from build123d import *

# Parameters (mm, degrees)
ESQUISSE1_W        = 400
ESQUISSE1_H        = 100
ESQUISSE1_W_2      = 395
ESQUISSE1_H_2      = 95
BOSS_EXTRU_2_DEPTH = 100
ESQUISSE3_W        = 400
ESQUISSE3_H        = 100
ESQUISSE3_W_2      = 380
ESQUISSE3_H_2      = 80
BOSS_EXTRU_3_DEPTH = 25
BOSS_EXTRU_4_START = 100
ESQUISSE4_W        = 70
ESQUISSE4_H        = 25
ESQUISSE4_W_2      = 25
ESQUISSE4_H_2      = 70
BOSS_EXTRU_4_DEPTH = 10


with BuildPart() as part:
    # Esquisse1 → Boss.-Extru.2 (new body)
    with BuildSketch(Plane.XY):
        Rectangle(ESQUISSE1_W, ESQUISSE1_H)
        Rectangle(ESQUISSE1_W_2, ESQUISSE1_H_2, mode=Mode.SUBTRACT)
    extrude(amount=BOSS_EXTRU_2_DEPTH)

    # Esquisse3 → Boss.-Extru.3 (add)
    with BuildSketch(Plane.XY):
        Rectangle(ESQUISSE3_W, ESQUISSE3_H)
        Rectangle(ESQUISSE3_W_2, ESQUISSE3_H_2, mode=Mode.SUBTRACT)
    extrude(amount=BOSS_EXTRU_3_DEPTH)

    # Esquisse4 → Boss.-Extru.4 (add)
    with BuildSketch(Plane.XY.offset(BOSS_EXTRU_4_START)):
        with Locations((-235, 0)):
            Rectangle(ESQUISSE4_W, ESQUISSE4_H)
        with Locations((235, 0)):
            Rectangle(ESQUISSE4_W, ESQUISSE4_H)
        with Locations((-141.037105637, 85)):
            Rectangle(ESQUISSE4_W_2, ESQUISSE4_H_2)
        with Locations((141.037105637, 85)):
            Rectangle(ESQUISSE4_W_2, ESQUISSE4_H_2)
        with Locations((-66.58352445, 85)):
            Rectangle(ESQUISSE4_W_2, ESQUISSE4_H_2)
        with Locations((66.58352445, 85)):
            Rectangle(ESQUISSE4_W_2, ESQUISSE4_H_2)
        with Locations((141.037105637, -85)):
            Rectangle(ESQUISSE4_W_2, ESQUISSE4_H_2)
        with Locations((66.58352445, -85)):
            Rectangle(ESQUISSE4_W_2, ESQUISSE4_H_2)
        with Locations((-66.58352445, -85)):
            Rectangle(ESQUISSE4_W_2, ESQUISSE4_H_2)
        with Locations((-141.037105637, -85)):
            Rectangle(ESQUISSE4_W_2, ESQUISSE4_H_2)
    extrude(amount=-BOSS_EXTRU_4_DEPTH)


solid = part.part
Can you work these out from the model? Positions are in its coordinate system, mm. A direction names the side the tool comes from. Coordinates: 2 decimals unless noted, no trailing zeros. Write each loop counter-clockwise with the first axis right and the second up, starting at its lowest first coordinate (ties: lowest second). Pieces come first, ordered by that corner, then holes.
Q1. Imagine slicing it at A-A, the plane y = -79.5. List the corners of the cut face in (x, z) for me, plus the area to 3 significant figures.
Results found:
outline: (-153.54, 90) - (-128.54, 90) - (-128.54, 100) - (-153.54, 100) - close; (-79.08, 90) - (-54.08, 90) - (-54.08, 100) - (-79.08, 100) - close; (54.08, 90) - (79.08, 90) - (79.08, 100) - (54.08, 100) - close; (128.54, 90) - (153.54, 90) - (153.54, 100) - (128.54, 100) - close
area: 1,000 mm2
Q2. For P1, Ø20, axis at x = 68.5, y = 87.5, coming from the -Z side; P2, Ø11, axis at y = -76, z = 93, coming from the +X side; P3, Ø1, axis at y = 5.5, z = 33.5, coming from the -X side, each with a flat end and sliding along its axis, tell me the tip position at first contact or that it passes through.
Results found:
P1: stops at z = 90
P2: stops at x = 153.54
P3: stops at x = -200
Q3. Please list where these lines run through material, in increasing order: L1, parallel to Y at x = 116, z = 80.5; L2, parallel to X at y = -38, z = 84; L3, parallel to X at y = -25, z = 13.
Results found:
L1: y = -50 to -47.5, 47.5 to 50
L2: x = -200 to -197.5, 197.5 to 200
L3: x = -200 to -190, 190 to 200
Q4. Imagine slicing it at C-C, the plane x = 160. List the corners of the cut face in (y, z) for me, plus the area to 3 significant figures.
Results found:
outline: (-50, 0) - (-40, 0) - (-40, 25) - (-47.5, 25) - (-47.5, 100) - (-50, 100) - close; (40, 0) - (50, 0) - (50, 100) - (47.5, 100) - (47.5, 25) - (40, 25) - close
area: 875 mm2
Q5. If we mould it in two halves opening along Y, with no side actions, what happens to faces 6 (the face through (-200, -1, 49)), 7 (the face through (-3, 40, 12)), 8 (the face through (235, -12.5, 95)), 9 (the face through (-67, 120, 95))? For each: +Y half, -Y half, draft (parallel to the pull), parting line (faces both ways), or undercut.
Results found:
face 6: draft
face 7: undercut
face 8: -Y half
face 9: +Y half
Q6. Which directions (+Z, -Z, +X, -X, +Y, -Y) give clear straight access to the entire face, cutting with the end or side of a thin tool? Please do faces 1 (the face through (-67, -85, 90)), 2 (the face through (-141, 85, 90)), 3 (the face through (-190, -1, 12)), 4 (the face through (54.084, 85, 95)), 5 (the face through (-153.537, -85, 95)).
Results found:
face 1: -Z, +X, -X, -Y
face 2: -Z, +X, -X, +Y
face 3: +Z, -Z
face 4: +Z, -Z, +Y
face 5: +Z, -Z, -X, -Y
Q7. Imagine slicing it at B-B, the plane z = 38. List the corners of the cut face in (x, y) for me.
Results found:
outline: (-200, -50) - (200, -50) - (200, 50) - (-200, 50) - close; hole (-197.5, -47.5) - (197.5, -47.5) - (197.5, 47.5) - (-197.5, 47.5) - close
Q8. Imagine slicing it at D-D, the plane y = 28. List the corners of the cut face in (x, z) for me.
Results found:
outline: (-200, 0) - (-190, 0) - (-190, 25) - (-197.5, 25) - (-197.5, 100) - (-200, 100) - close; (190, 0) - (200, 0) - (200, 100) - (197.5, 100) - (197.5, 25) - (190, 25) - close
